Build history of the part. All positions in model axes, mm. Face numbers are marked on the shaded views. Round coordinates to 2 decimals unless told otherwise and drop trailing zeros. Write each loop counter-clockwise with the first axis right and the second up, starting at its lowest first coordinate (ties: lowest second). Pieces come first, ordered by that corner, then holes.
Item 1: Band-saw the part on A-A, the plane z = -2.75. Count the separate pieces of the cut face and the enclosed holes in it, then the cut area to 3 significant figures.
Item 2: Wall check: probe 1 along X at (y, z) = (-30, -8.5); probe 2 along Z at (x, y) = (19.5, -1); probe 3 along Z at (x, y) = (16.5, 14.5). Give the ranges that are in metal, low to high.
Item 3: Mould opens along X. For the marked faces 1, 2 and 3 say: +X half, -X half, draft (parallel to the pull), parting line (faces both ways), or undercut.
Item 4: Band-saw the part on B-B, the plane y = -21.5. Write the cut outline in (x, z), then the cut area to 3 significant figures.
Item 5: Drop flat-ended pins along their axis: pin 1 Ø2 at (x, y) = (13, -6.5) entering from -Z; pin 2 Ø8 at (x, z) = (3, -7) entering from -Y; pin 3 Ø0.9 at (x, y) = (-6.5, 33) entering from -Z; pin 4 Ø5 at (y, z) = (-19.5, -3) entering from +X. Give the stop position or say it passes through.
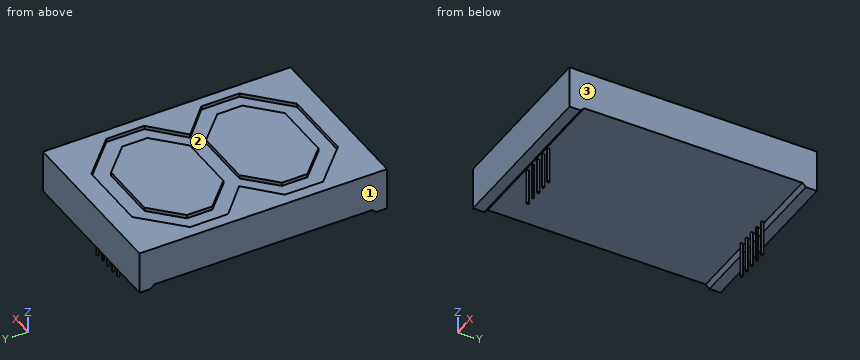
Autodesk Inventor part; units mm, degrees
ref_plane "YZ Plane" through (0, 0, 0) normal (1, 0, 0) x (0, 1, 0)
ref_plane "XZ Plane" through (0, 0, 0) normal (0, 1, 0) x (-1, 0, 0)
ref_plane "XY Plane" through (0, 0, 0) normal (0, 0, 1) x (1, 0, 0)
sketch "Sketch1" plane through (0, 0, 0) normal (0, 0, 1) x (1, 0, 0)
  line L0 (-23.9, 34.85) -> (23.9, 34.85)
  line L1 (23.9, 34.85) -> (23.9, -34.85)
  line L2 (23.9, -34.85) -> (-23.9, -34.85)
  line L3 (-23.9, -34.85) -> (-23.9, 34.85)
  dimension "d0" = 47.8
  dimension "d1" = 69.7
extrude "Extrusion1" add sketch "Sketch1" along normal blind 11
sketch "Sketch2" plane through (0, 0, 0) normal (0, 0, -1) x (-1, 0, 0)
  line L0 (-23.9, 34.85) -> (23.9, 34.85)
  line L1 (23.9, 34.85) -> (23.9, -34.85)
  line L2 (-23.9, 34.85) -> (23.9, 34.85)
  line L3 (23.9, 34.85) -> (23.9, 31.7132)
  line L4 (23.9, 31.7132) -> (-23.9, 31.7132)
  line L5 (-23.9, 31.7132) -> (-23.9, 34.85)
  line L6 (23.9, -34.85) -> (-23.9, -34.85)
  line L7 (-23.9, -34.85) -> (-23.9, 34.85)
  line L8 (23.9, -34.85) -> (-23.9, -34.85)
  line L9 (-23.9, -34.85) -> (-23.9, -31.7132)
  line L10 (-23.9, -31.7132) -> (23.9, -31.7132)
  line L11 (23.9, -31.7132) -> (23.9, -34.85)
  line L12 (-23.9, 34.85) -> (23.9, 34.85)
  line L13 (23.9, 34.85) -> (23.9, 31.7132)
  line L14 (23.9, 31.7132) -> (-23.9, 31.7132)
  line L15 (-23.9, 31.7132) -> (-23.9, 34.85)
  line L16 (-23.9, -31.7132) -> (23.9, -31.7132)
  line L17 (23.9, -31.7132) -> (23.9, -34.85)
  line L18 (23.9, -34.85) -> (-23.9, -34.85)
  line L19 (-23.9, -34.85) -> (-23.9, -31.7132)
  point P0 (0, 0)
  dimension "d4" = 3.1368
  dimension "d5" = 3.1368
extrude "Extrusion2" add sketch "Sketch2" along normal blind 1 contours L0 L1 L4 L5 | L10 L1 L6 L7
chamfer "Chamfer1" distance 1 distance2 1 1 edges at (0, 31.7132, 0) measured on face at (-7.9667, -10.5711, 0)
chamfer "Chamfer2" distance 1 distance2 1 1 edges at (0, -31.7132, 0) measured on face at (-7.9667, -10.9042, 0)
sketch "Sketch3" plane through (0, 0, 0) normal (0, 0, -1) x (-1, 0, 0)
  circle A0 centre (0, 30.1) radius 0.3
  circle A1 centre (2.54, 30.1) radius 0.3
  circle A2 centre (5.08, 30.1) radius 0.3
  line L0 (-23.9, 30.7132) -> (23.9, 30.7132)
  line L1 (0, 30.7132) -> (0, 27.4639)
  circle A3 centre (-2.54, 30.1) radius 0.3
  circle A4 centre (-5.08, 30.1) radius 0.3
  line L2 (-5.649, 0) -> (7.1976, 0)
  circle A5 centre (0, -30.1) radius 0.3
  circle A6 centre (2.54, -30.1) radius 0.3
  circle A7 centre (5.08, -30.1) radius 0.3
  circle A8 centre (-2.54, -30.1) radius 0.3
  circle A9 centre (-5.08, -30.1) radius 0.3
  point P0 (0, 0)
  dimension "d14" = 0.6
  dimension "d15" = 0.6
  dimension "d16" = 0.6
extrude "Extrusion3" add sketch "Sketch3" along normal blind 10
sketch "Sketch4" plane through (0, 0, 11) normal (0, 0, 1) x (1, 0, 0)
  line L0 (-28.3117, 29.0487) -> (26.925, 29.0487) construction
  line L1 (26.925, 29.0487) -> (26.925, -28.8882) construction
  line L2 (26.925, -28.8882) -> (-28.3117, -28.8882) construction
  line L3 (-28.3117, -28.8882) -> (-28.3117, 29.0487) construction
  line L4 (20.8139, -18.7031) -> (10.2024, -28.8882)
  line L5 (10.2024, -28.8882) -> (-10.0732, -28.8882)
  line L6 (-10.0732, -28.8882) -> (-20.6373, -18.7031)
  line L7 (-20.6373, -18.7031) -> (-20.6373, -7.9494)
  line L8 (-20.6373, -7.9494) -> (-12.0628, 0.0566)
  line L9 (-12.0628, 0.0566) -> (-20.6373, 8.0626)
  line L10 (-20.6373, 8.0626) -> (-20.6373, 18.7688)
  line L11 (-20.6373, 18.7688) -> (-10.0732, 29.0487)
  line L12 (-10.0732, 29.0487) -> (10.155, 29.0487)
  line L13 (10.155, 29.0487) -> (20.8139, 18.7688)
  line L14 (20.8139, 18.7688) -> (20.8139, 8.0626)
  line L15 (20.8139, 8.0626) -> (12.192, 0.0566)
  line L16 (12.192, 0.0566) -> (20.8139, -7.9968)
  line L17 (20.8139, -7.9968) -> (20.8139, -18.7031)
  line L18 (16.124, -16.9029) -> (16.124, -9.797)
  line L19 (16.124, -9.797) -> (8.3075, -2.2173)
  line L20 (8.3075, -2.2173) -> (-8.2256, -2.2173)
  line L21 (-8.2256, -2.2173) -> (-15.9948, -9.7496)
  line L22 (-15.9948, -9.7496) -> (-15.9948, -16.9029)
  line L23 (-15.9948, -16.9029) -> (-8.2256, -24.4352)
  line L24 (-8.2256, -24.4352) -> (8.3075, -24.4352)
  line L25 (8.3075, -24.4352) -> (16.124, -16.9029)
  line L26 (16.124, 9.8627) -> (16.124, 16.9687)
  line L27 (16.124, 16.9687) -> (8.3075, 24.5483)
  line L28 (8.3075, 24.5483) -> (-8.2256, 24.5483)
  line L29 (-8.2256, 24.5483) -> (-15.9948, 17.016)
  line L30 (-15.9948, 17.016) -> (-15.9948, 9.8627)
  line L31 (-15.9948, 9.8627) -> (-8.2256, 2.3305)
  line L32 (-8.2256, 2.3305) -> (8.3075, 2.3305)
  line L33 (8.3075, 2.3305) -> (16.124, 9.8627)
  point P0 (0, 0)
extrude "Extrusion4" cut sketch "Sketch4" against normal blind 1
properties part number "Digit"
Results:
1. separate pieces: 10
1. enclosed holes: 0
1. area: 2.83 mm2
2. probe 1: x = -5.36 to -4.8, -2.82 to -2.26, -0.28 to 0.28, 2.26 to 2.82, 4.8 to 5.36
2. probe 2: z = 0 to 11
2. probe 3: z = 0 to 10
3. face 1: -X half
3. face 2: undercut
3. face 3: +X half
4. outline: (-23.9, 0) - (23.9, 0) - (23.9, 11) - (17.9, 11) - (17.9, 10) - (11.35, 10) - (11.35, 11) - (-11.25, 11) - (-11.25, 10) - (-17.74, 10) - (-17.74, 11) - (-23.9, 11) - close
4. area: 513 mm2
5. pin 1: stops at z = 0
5. pin 2: stops at y = -30.4
5. pin 3: stops at z = -1
5. pin 4: passes through
